Input: part model. Units: mm. Frame: model coordinates. A direction names the side the tool comes from. Round coordinates to 2 decimals unless told otherwise and drop trailing zeros. Write each loop counter-clockwise with the first axis right and the second up, starting at its lowest first coordinate (ties: lowest second). Pieces come first, ordered by that corner, then holes. Notation, with made-up numbers: (46.25, 2) - (77.25, 2) arc R18 ccw to (77.25, 20) - close; hole circle Ø4 at (24.5, -12.5). An arc over 180 degrees is marked (long way). Use one line per item in the form item = value.
Autodesk Inventor part; units mm, degrees
ref_plane "YZ Plane" through (0, 0, 0) normal (1, 0, 0) x (0, 1, 0)
ref_plane "XZ Plane" through (0, 0, 0) normal (0, 1, 0) x (-1, 0, 0)
ref_plane "XY Plane" through (0, 0, 0) normal (0, 0, 1) x (1, 0, 0)
sketch "Sketch2" plane through (0, 0, 0) normal (0, 1, 0) x (-1, 0, 0)
  line L0 (-47.625, 80.645) -> (47.625, 80.645)
  line L1 (47.625, 80.645) -> (47.625, -80.645)
  line L2 (47.625, -80.645) -> (-47.625, -80.645)
  line L3 (-47.625, -80.645) -> (-47.625, 80.645)
  line L4 (-47.625, 80.645) -> (47.625, -80.645) construction
  line L5 (47.625, 80.645) -> (-47.625, -80.645) construction
  point P0 (0, 0)
  dimension "d6" = 161.29
  dimension "d7" = 95.25
extrude "Extrusion2" add sketch "Sketch2" along normal blind 6.35
sketch "Sketch3" plane through (0, 6.35, 0) normal (0, 1, 0) x (1, 0, 0)
  line L0 (47.625, 80.645) -> (-47.625, 80.645)
  line L1 (47.625, -80.645) -> (-47.625, -80.645)
  line L2 (-47.625, -80.645) -> (-47.625, 80.645)
  line L3 (-47.625, 80.645) -> (47.625, 80.645)
  line L4 (47.625, 80.645) -> (47.625, -80.645)
  line L5 (47.625, -80.645) -> (-47.625, 80.645) construction
  line L6 (-47.625, -80.645) -> (47.625, 80.645) construction
  line L7 (41.275, -74.295) -> (-41.275, -74.295)
  line L8 (-41.275, -74.295) -> (-41.275, 74.295)
  line L9 (-41.275, 74.295) -> (41.275, 74.295)
  line L10 (41.275, 74.295) -> (41.275, -74.295)
  line L11 (41.275, -74.295) -> (-41.275, 74.295) construction
  line L12 (-41.275, -74.295) -> (41.275, 74.295) construction
  point P0 (0, 0)
  dimension "d10" = 148.59
  dimension "d11" = 82.55
extrude "Extrusion3" add sketch "Sketch3" along normal blind 31.75
sketch "Sketch6" plane through (0, 38.1, 0) normal (0, 1, 0) x (1, 0, 0)
  line L0 (44.45, -77.47) -> (-44.45, -77.47)
  line L1 (-44.45, -77.47) -> (-44.45, 77.47)
  line L2 (-44.45, 77.47) -> (44.45, 77.47)
  line L3 (44.45, 77.47) -> (44.45, -77.47)
  line L4 (44.45, -77.47) -> (-44.45, 77.47) construction
  line L5 (-44.45, -77.47) -> (44.45, 77.47) construction
  point P0 (0, 0)
  dimension "d29" = 154.94
  dimension "d30" = 88.9
extrude "Extrusion6" cut sketch "Sketch6" against normal blind 4.7625
sketch "Sketch9" plane through (-47.625, 0, -80.645) normal (-1, 0, 0) x (0, 0, 1)
  line L0 (161.29, 0) -> (0, 0)
  line L1 (74.8462, 0) -> (81.1962, 0)
  line L2 (81.1962, 0) -> (81.1962, 4.1295)
  line L3 (81.1962, 4.1295) -> (74.8462, 4.1295)
  line L4 (74.8462, 4.1295) -> (74.8462, 0)
  point P0 (80.645, 0)
  dimension "d57" = 6.35
extrude "Extrusion9" add sketch "Sketch9" along normal blind 25.4
sketch "Sketch10" plane through (-47.625, 0, 80.645) normal (0, 0, 1) x (1, 0, 0)
  line L0 (95.25, 0) -> (0, 0)
  line L1 (39.3541, 0) -> (45.7041, 0)
  line L2 (45.7041, 0) -> (45.7041, 3.778)
  line L3 (45.7041, 3.778) -> (39.3541, 3.778)
  line L4 (39.3541, 3.778) -> (39.3541, 0)
  point P0 (47.625, 0)
  dimension "d56" = 6.35
extrude "Extrusion10" add sketch "Sketch10" along normal blind 25.4
sketch "Sketch11" plane through (47.625, 0, 80.645) normal (1, 0, 0) x (0, 0, -1)
  line L0 (161.29, 0) -> (0, 0)
  line L1 (86.4438, 4.1295) -> (86.4438, 0)
  line L2 (80.0938, 0) -> (86.4438, 0)
  line L3 (86.4438, 0) -> (86.4438, 4.1295)
  line L4 (86.4438, 4.1295) -> (80.0938, 4.1295)
  line L5 (80.0938, 4.1295) -> (80.0938, 0)
  point P0 (80.645, 0)
  dimension "d55" = 6.35
extrude "Extrusion11" add sketch "Sketch11" along normal blind 25.4
sketch "Sketch12" plane through (47.625, 0, -80.645) normal (0, 0, -1) x (-1, 0, 0)
  line L0 (41.275, 0) -> (47.625, 0)
  line L1 (47.625, 0) -> (47.625, 3.778)
  line L2 (47.625, 3.778) -> (41.275, 3.778)
  line L3 (41.275, 3.778) -> (41.275, 0)
  dimension "d54" = 6.35
extrude "Extrusion12" add sketch "Sketch12" along normal blind 25.4
fillet "Fillet1" radius 3.175 12 edges at (47.625, 19.05, 80.645) (47.625, 19.05, -80.645) (-47.625, 19.05, -80.645) (-47.625, 19.05, 80.645) (44.45, 35.7187, -77.47) (41.275, 19.8437, -74.295) (-41.275, 19.8437, -74.295) (-44.45, 35.7187, -77.47) (-41.275, 19.8437, 74.295) (-44.45, 35.7187, 77.47) (41.275, 19.8437, 74.295) (44.45, 35.7187, 77.47)
sketch "Sketch13" plane through (0, 0, 0) normal (0, -1, 0) x (1, 0, 0)
  line L0 (-24.765, 53.975) -> (24.765, 53.975) construction
  line L1 (24.765, 53.975) -> (24.765, -53.975) construction
  line L2 (24.765, -53.975) -> (-24.765, -53.975) construction
  line L3 (-24.765, -53.975) -> (-24.765, 53.975) construction
  line L4 (-24.765, 53.975) -> (24.765, -53.975) construction
  line L5 (24.765, 53.975) -> (-24.765, -53.975) construction
  circle A0 centre (24.765, 53.975) radius 10.9982
  circle A1 centre (24.765, 22.225) radius 10.9982
  circle A2 centre (24.765, -22.225) radius 10.9982
  circle A3 centre (24.765, -53.975) radius 10.9982
  line L6 (-47.625, -5.7988) -> (-47.625, -77.47) construction
  point P0 (0, 0)
  dimension "d58" = 21.9964
  dimension "d59" = 21.9964
  dimension "d60" = 21.9964
  dimension "d61" = 21.9964
  dimension "d62" = 31.75
  dimension "d63" = 44.45
  dimension "d64" = 31.75
  dimension "d66" = 72.39
extrude "Extrusion13" cut sketch "Sketch13" against normal up to next
properties part number "iceTubeClockBase"
(1) Cut plane A-A on y = 29.5. Output: boundary loops of the cut face in (x, z) (3 decimals), then the cut area to 3 significant figures.
Derived:
outline = (-47.625, -77.47) arc R3.175 ccw to (-44.45, -80.645) - (44.45, -80.645) arc R3.175 ccw to (47.625, -77.47) - (47.625, 77.47) arc R3.175 ccw to (44.45, 80.645) - (-44.45, 80.645) arc R3.175 ccw to (-47.625, 77.47) - close; hole (-41.275, -71.12) arc R3.175 ccw to (-38.1, -74.295) - (38.1, -74.295) arc R3.175 ccw to (41.275, -71.12) - (41.275, 71.12) arc R3.175 ccw to (38.1, 74.295) - (-38.1, 74.295) arc R3.175 ccw to (-41.275, 71.12) - close
area = 3,100 mm^2
(2) First-contact query: pin 1 Ø7 at (x, z) = (3.5, -98) entering from +Y; pin 2 Ø1.1 at (y, z) = (2, 99.5) entering from -X; pin 3 Ø19 at (y, z) = (25.5, 3.5) entering from -X (3 decimals). Flat tips, straight axial feed; report the tip coordinate or a pass-through.
Derived:
pin_1 = 3.78
pin_2 = -8.27
pin_3 = -47.625
(3) Access query for faces 5 (the face through (16.04, 3.13, -60.67)), 6 (the face through (1, 20, 74.295)), 7 (the face through (60, 2, -5.799)), 8 (the face through (60, 4.13, -3)). Directions: +Z, -Z, +X, -X, +Y, -Y. A direction counts if a zero-diameter tool reaches every point of the face in a straight line with its end or side. Return the directions, or none.
Derived:
face_5 = +Y, -Y
face_6 = +Y
face_7 = -Z, +X, +Y, -Y
face_8 = +Z, -Z, +X, +Y
(4) Draft query along Z for faces 1 (the face through (-44.45, 36, 1)), 2 (the face through (-60, 2, 0.551)), 3 (the face through (73.025, 2, -3)), 4 (the face through (44.45, 36, -1)). Return one class per face: released by +Z, released by -Z, zero draft, split by the parting line, or undercut.
Derived:
face_1 = undercut
face_2 = released by +Z
face_3 = zero draft
face_4 = undercut
(5) Cut plane D-D on x = -51.5. Output: boundary loops of the cut face in (y, z), then the cut area to 3 significant figures.
Derived:
outline = (0, -5.8) - (4.13, -5.8) - (4.13, 0.55) - (0, 0.55) - close
area = 26.2 mm^2
(6) Material intervals for L1, parallel to X at y = 20, z = 71 (3 decimals); L2, parallel to X at y = 35.5, z = 70.5 (3 decimals); L3, parallel to Z at x = 15, y = 7.5 (3 decimals), sorted ascending.
Derived:
L1 = -47.625 to -41.275, 41.275 to 47.625
L2 = -47.625 to -44.45, 44.45 to 47.625
L3 = -80.645 to -74.295, 74.295 to 80.645
